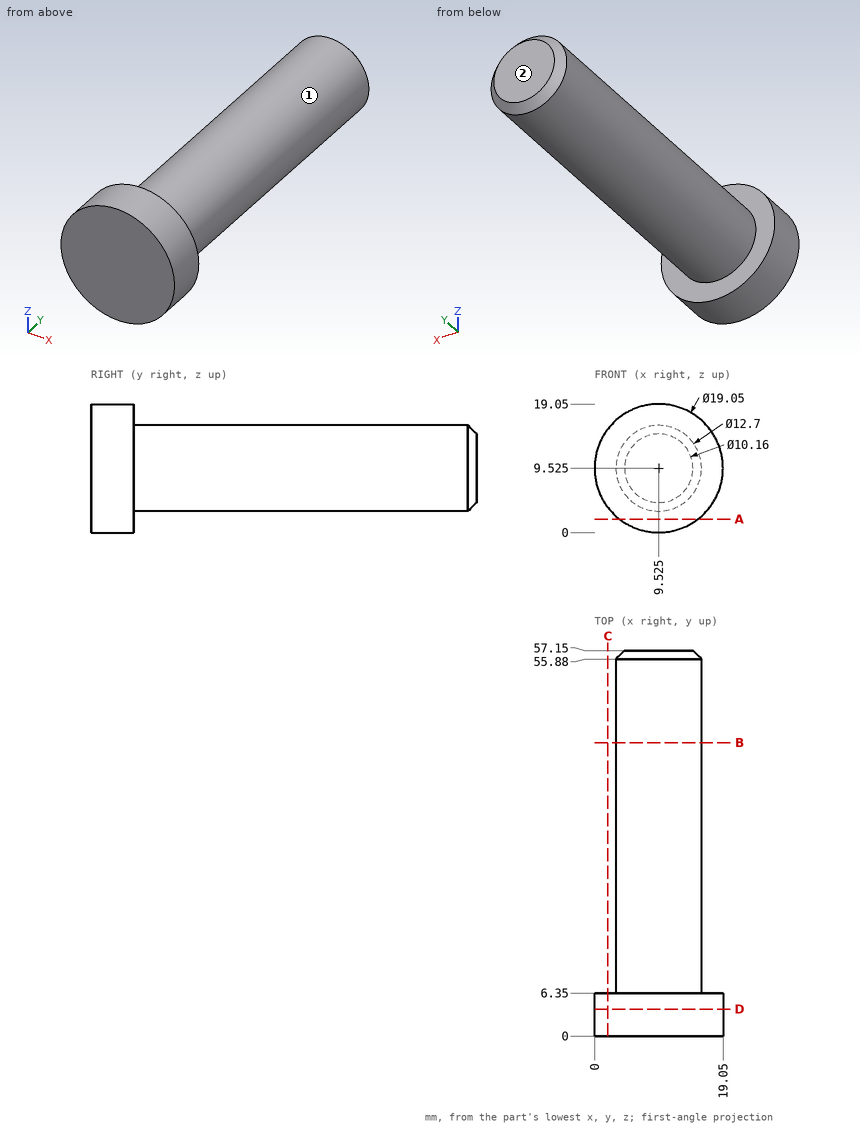
Geometry check sheet. Reference: drawing and pictorial views, mm from the part's lowest x, y, z. A direction names the side the tool comes from. Round coordinates to 2 decimals unless told otherwise and drop trailing zeros. Loops run counter-clockwise (first coordinate to the right, second up) from the corner with the lowest first, then second, coordinate; pieces in that order, holes last. Notation, with made-up numbers: (28.25, 68) - (41.25, 68) arc R26 ccw to (41.25, 103) - close; hole circle Ø8 at (-34.5, 61). An arc over 180 degrees is marked (long way). Use a Markdown table: item, result. Add a question column.
1. Section check A-A, the plane z = 2. Record the boundary of the cut face in (x, y).
2. Section check B-B, the plane y = 43.5. Record the boundary of the cut face in (x, z) (3 decimals), plus the area to 3 significant figures.
3. Section check C-C, the plane x = 2. Record the boundary of the cut face in (y, z).
4. Section check D-D, the plane y = 4. Record the boundary of the cut face in (x, z) (3 decimals), plus the area to 3 significant figures.
5. Thickness scan on probe 1 along Y at (x, z) = (10.5, 2.5); probe 2 along X at (y, z) = (4, 8); probe 3 along Z at (x, y) = (8.5, 16). Record the ranges inside material, lowest first. Write a range as [from, to].
6. Gauge pin test, flat ends, axial feed: pin 1 (6 mm diameter, centred on x = 9, z = 9.5, fed in from -Y); pin 2 (6 mm diameter, centred on x = 5, y = 5.5, fed in from +Z); pin 3 (3 mm diameter, centred on y = 46.5, z = 6, fed in from -X); pin 4 (2 mm diameter, centred on x = 13.5, y = 22, fed in from -Z) (3 decimals). Record the tip position at first contact, or that the pin passes through.
7. Access from +Z, -Z, +X, -X, +Y, -Y to the whole of each face (thin tool, end or side, straight path). Record for the marked faces 1 and 2.
Checks:
| question | item | result |
|---|---|---|
| 1 | outline | (3.69, 0) - (15.36, 0) - (15.36, 6.35) - (3.69, 6.35) - close |
| 2 | outline | circle Ø12.7 at (9.525, 9.525) |
| 2 | area | 127 mm^2 |
| 3 | outline | (0, 3.69) - (6.35, 3.69) - (6.35, 15.36) - (0, 15.36) - close |
| 4 | outline | circle Ø19.05 at (9.525, 9.525) |
| 4 | area | 285 mm^2 |
| 5 | probe 1 | y = [0, 6.35] |
| 5 | probe 2 | x = [0.12, 18.93] |
| 5 | probe 3 | z = [3.26, 15.79] |
| 6 | pin 1 | stops at y = 0 |
| 6 | pin 2 | stops at z = 18.93 |
| 6 | pin 3 | stops at x = 3.51 |
| 6 | pin 4 | stops at z = 3.915 |
| 7 | face 1 | +Y |
| 7 | face 2 | +Z, -Z, +X, -X, +Y |
